Answer from the drawing. Dimensions are ordinates in mm from the lowest x, y and z of the part. Round coordinates to 2 decimals unless told otherwise and drop trailing zeros. Order: outer loops, then holes, each group sorted by start corner. A loop starts at its lowest first (then second) coordinate and runs counter-clockwise, first axis right, second up.
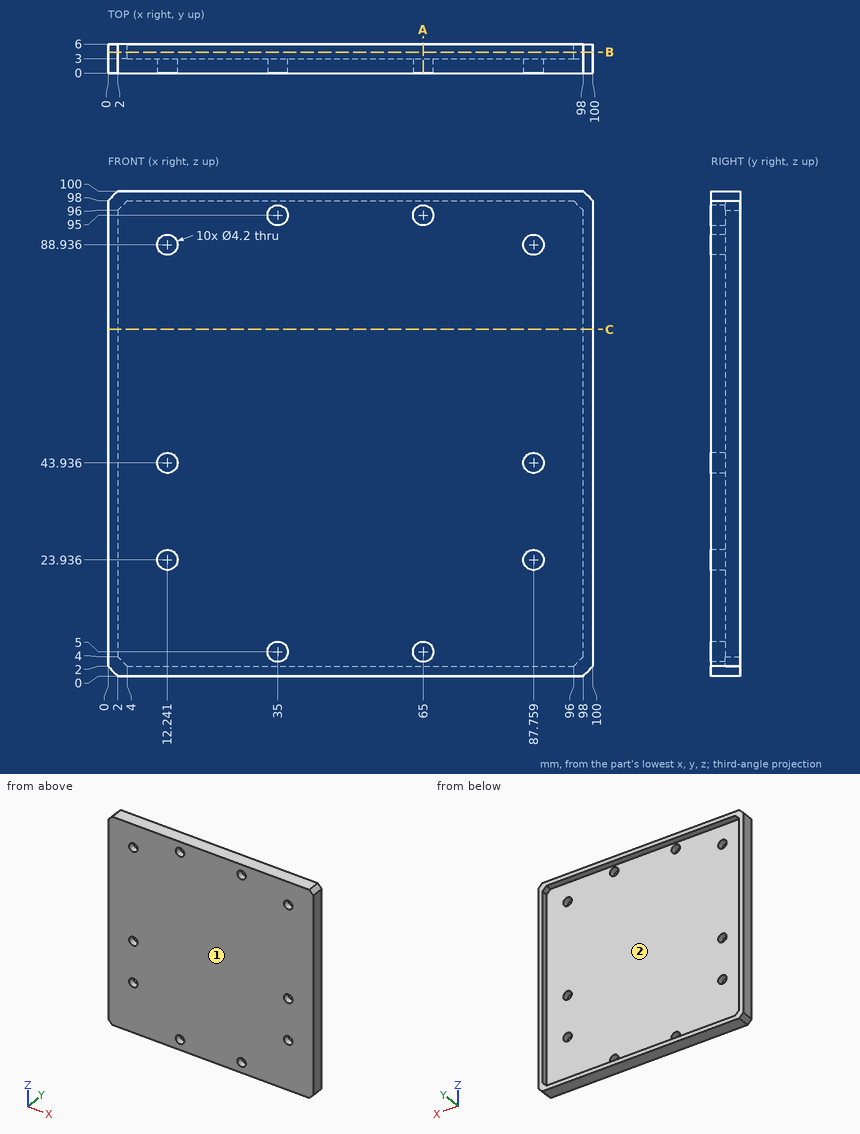
Q1. A cutting plane is placed at C-C, the plane z = 71.5. Give the vertices of the cut face in (x, y).
Outcome:
outline: (0, 0) - (100, 0) - (100, 6) - (98, 6) - (98, 3) - (2, 3) - (2, 6) - (0, 6) - close
Q2. Straight lines are drawn through the part: probe 1 along Z at (x, y) = (65, 1.9); probe 2 along X at (y, z) = (1.85, 95); probe 3 along Z at (x, y) = (20, 5.2). For each, find the intervals that lie inside material, in ascending order.
Outcome:
probe 1: z = 0 to 2.9, 7.1 to 92.9, 97.1 to 100
probe 2: x = 0 to 32.9, 37.1 to 62.9, 67.1 to 100
probe 3: z = 0 to 2, 98 to 100
Q3. A cutting plane is placed at B-B, the plane y = 4.3. Give the vertices of the cut face in (x, z).
Outcome:
outline: (0, 2) - (2, 0) - (98, 0) - (100, 2) - (100, 98) - (98, 100) - (2, 100) - (0, 98) - close; hole (2, 4) - (4, 2) - (96, 2) - (98, 4) - (98, 96) - (96, 98) - (4, 98) - (2, 96) - close
Q4. A cutting plane is placed at A-A, the plane x = 65. Give the vertices of the cut face in (y, z).
Outcome:
outline: (0, 0) - (6, 0) - (6, 2) - (3, 2) - (3, 2.9) - (0, 2.9) - close; (0, 7.1) - (3, 7.1) - (3, 92.9) - (0, 92.9) - close; (0, 97.1) - (3, 97.1) - (3, 98) - (6, 98) - (6, 100) - (0, 100) - close
Q5. For a pull along Z with two mould halves and no side action, classify the marked faces 1 and 2 as released by +Z, released by -Z, zero draft, split by the parting line, or undercut.
Outcome:
face 1: zero draft
face 2: undercut
Q6. A flat-ended cylindrical pin translates along its axis: pin 1 (4 mm diameter, centred on x = 72, z = 87, fed in from +Y). Find the tip coordinate at first contact, or state that the pin passes through.
Outcome:
pin 1: stops at y = 3
